Input: dimensioned drawing with shaded views. Units: mm. Origin: part minimum x, y, z. Coordinates: 2 decimals unless noted, no trailing zeros. Order: outer loops, then holes, each group sorted by start corner. A loop starts at its lowest first (then second) coordinate and runs counter-clockwise, first axis right, second up. Notation, with made-up numbers: M -19.5,-4 L 6.5,-4 A36 cw 6.5,32 Z; hole C -5.75,68 d7. An arc over 180 degrees is marked long. Use CSV: the item, a comma, the result in double quotes. Start each with the question number.
1. Material intervals for line 1 (Z direction, x = 5.5, y = 7); line 2 (Z direction, x = 0.5, y = 3); line 3 (Y direction, x = 0.5, z = 3.5), sorted ascending.
2. Section query A-A on z = 7. Return the cut outline in (x, y), and give its area (3 significant figures).
3. First-contact query: P1, Ø2, axis at y = 4.5, z = 6.5, coming from the -X side; P2, Ø1, axis at x = 6.5, z = 8, coming from the +Y side. Flat tips, straight axial feed; report the tip coordinate or a pass-through.
4. Section query C-C on x = 2. Return the cut outline in (y, z), and give its area (3 significant figures).
5. Pull-direction query (Z, two-part tool) for the marked faces 1, 2 and 3; classes: pulls with the +Z half, pulls with the -Z half, needs draft (parallel to the pull), parting line crosses it, or undercut.
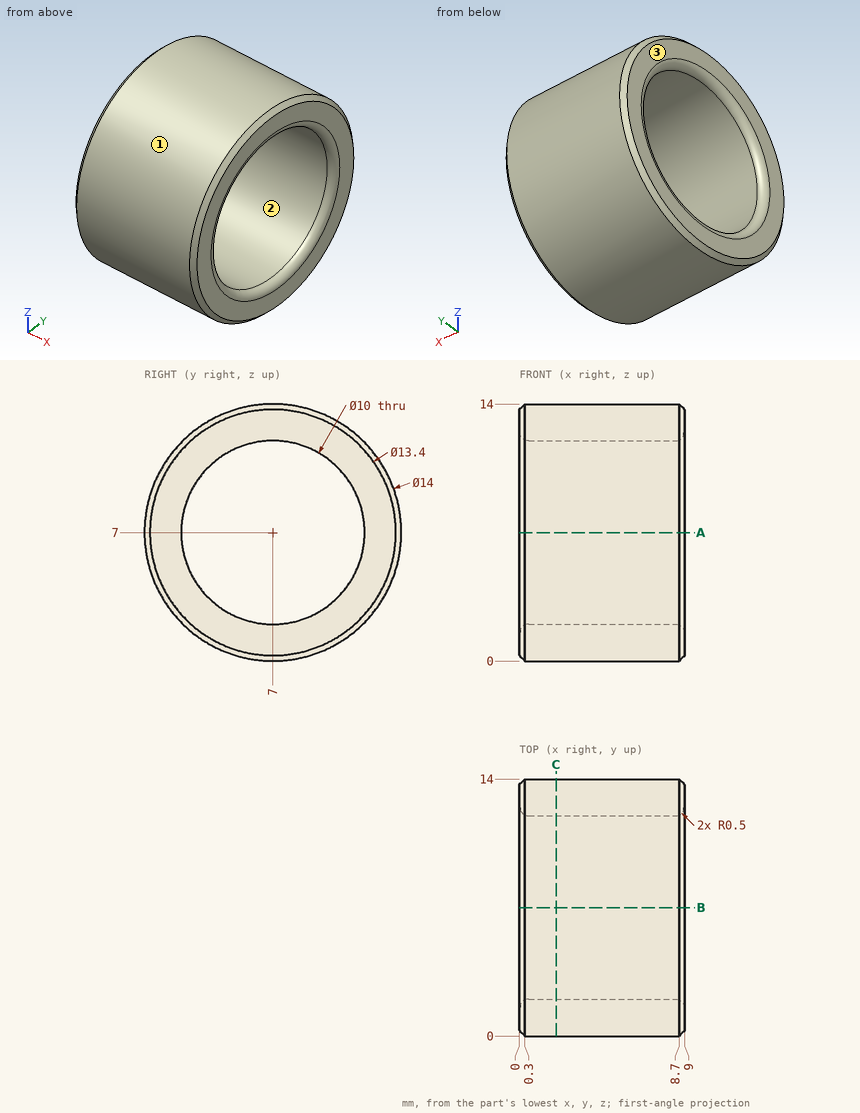
Results list:
1,line 1,"z = 0 to 2, 12 to 14"
1,line 2,"z = 1.26 to 4, 10 to 12.74"
1,line 3,"y = 0.94 to 3.43, 10.57 to 13.06"
2,outline,"M 0,0.3 L 0.3,0 L 8.7,0 L 9,0.3 L 9,1.5 A0.5 ccw 8.5,2 L 0.5,2 A0.5 ccw 0,1.5 Z; M 0,12.5 A0.5 ccw 0.5,12 L 8.5,12 A0.5 ccw 9,12.5 L 9,13.7 L 8.7,14 L 0.3,14 L 0,13.7 Z"
2,area,"35.6 mm²"
3,P1,"passes through"
3,P2,"stops at y = 13.98"
4,outline,"C 7,7 d14; hole C 7,7 d10"
4,area,"75.4 mm²"
5,face 1,"parting line crosses it"
5,face 2,"undercut"
5,face 3,"needs draft"
